Part model, mm, in its own coordinate system. A direction names the side the tool comes from. Round coordinates to 2 decimals unless told otherwise and drop trailing zeros. Write each loop counter-clockwise with the first axis right and the second up, starting at its lowest first coordinate (ties: lowest second). Pieces come first, ordered by that corner, then holes. Notation, with made-up numbers: (-27, -29.75) -> (8, -29.75) arc R25 cw to (8, -14.75) -> close; hole circle Ø1 at (-27, -13). An arc over 180 degrees is marked (long way). Use CSV: the item, a comma, the result in double quotes. Start each with the question number.
(1) Saw through at A-A (z = 4.5). Give the cut face in (x, y).
(2) Which spindle directions (+Z, -Z, +X, -X, +Y, -Y) get a long thin tool onto all of the face, cutting with end or side? Do faces 1 (the flat face through (47.5, -1, -1)), 2 (the flat face through (21, -1, 32.121)). Say none if no direction does.
(3) Saw through at C-C (x = 26). Give the cut face in (y, z).
(4) Two-plate mould, pull along Z, no slides. Class faces 3 (the cylindrical face through (-45.09, -1.48, 45)), 4 (the flat face through (-1, 0, 1)), 5 (the cylindrical face through (-46.6, -1.48, 46.64)): released by +Z, released by -Z, zero draft, split by the parting line, or undercut.
(5) Saw through at D-D (y = -1.1). Count the separate pieces of the cut face and the enclosed holes in it, plus the area to 3 significant figures.
(6) Drop a flat-ended pin along its axis: pin 1 (3 mm diameter, centred on x = 43.95, z = -43.95, fed in from -Y). Give the stop position or say it passes through.
(7) Probe line 1 (X direction, y = -2.6, z = 27); line 2 (Z direction, x = -25.4, y = -2.05); line 3 (Z direction, x = -43.95, y = -1.8). List the from-to ranges inside material, lowest first. Write a range as [from, to].
(8) Saw through at B-B (x = 0). Give the cut face in (y, z).
```python
from build123d import *

# Parameters (mm, degrees)
F0_R     = 1.55
F0_R_2   = 3.8
F0_R_3   = 3
F0_W     = 22.7
F0_H     = 10.2
F1_DEPTH = 3


with BuildPart() as f1:
    # F0 (on Front) → F1 (new body)
    with BuildSketch(Plane.XZ):
        with BuildLine():
            Line((-44.5, -47.5), (44.5, -47.5))
            ThreePointArc((44.5, -47.5), (46.62132, -46.62132), (47.5, -44.5))
            Line((47.5, -44.5), (47.5, 44.5))
            ThreePointArc((47.5, 44.5), (46.62132, 46.62132), (44.5, 47.5))
            Line((44.5, 47.5), (-44.5, 47.5))
            ThreePointArc((-44.5, 47.5), (-46.62132, 46.62132), (-47.5, 44.5))
            Line((-47.5, 44.5), (-47.5, -44.5))
            ThreePointArc((-47.5, -44.5), (-46.62132, -46.62132), (-44.5, -47.5))
        make_face()
        with Locations((-43.95, -43.95)):
            Circle(F0_R, mode=Mode.SUBTRACT)
        with Locations((-25.4, -18.782858)):
            Circle(F0_R_2, mode=Mode.SUBTRACT)
        with Locations((43.95, -43.95)):
            Circle(F0_R, mode=Mode.SUBTRACT)
        with Locations((0, -18.782858)):
            Circle(F0_R_2, mode=Mode.SUBTRACT)
        with Locations((25.4, -18.782858)):
            Circle(F0_R_2, mode=Mode.SUBTRACT)
        with Locations((-21.6, 4.5)):
            Circle(F0_R_3, mode=Mode.SUBTRACT)
        with Locations((-43.95, 43.95)):
            Circle(F0_R, mode=Mode.SUBTRACT)
        with Locations((-21.6, 27.020905)):
            Rectangle(F0_W, F0_H, mode=Mode.SUBTRACT)
        with Locations((21.6, 4.5)):
            Circle(F0_R_3, mode=Mode.SUBTRACT)
        with Locations((21.6, 27.020905)):
            Rectangle(F0_W, F0_H, mode=Mode.SUBTRACT)
        with Locations((43.95, 43.95)):
            Circle(F0_R, mode=Mode.SUBTRACT)
    extrude(amount=F1_DEPTH)


solid = f1.part
```
Answers:
1,outline,"(-47.5, -3) -> (-24.6, -3) -> (-24.6, 0) -> (-47.5, 0) -> close; (-18.6, -3) -> (18.6, -3) -> (18.6, 0) -> (-18.6, 0) -> close; (24.6, -3) -> (47.5, -3) -> (47.5, 0) -> (24.6, 0) -> close"
2,face 1,"+Z, -Z, +X, +Y, -Y"
2,face 2,"+Y, -Y"
3,outline,"(-3, -47.5) -> (0, -47.5) -> (0, -22.54) -> (-3, -22.54) -> close; (-3, -15.03) -> (0, -15.03) -> (0, 21.92) -> (-3, 21.92) -> close; (-3, 32.12) -> (0, 32.12) -> (0, 47.5) -> (-3, 47.5) -> close"
4,face 3,"undercut"
4,face 4,"zero draft"
4,face 5,"released by +Z"
5,separate pieces,"1"
5,enclosed holes,"11"
5,area,"8,330 mm²"
6,pin 1,"passes through"
7,line 1,"x = [-47.5, -32.95], [-10.25, 10.25], [32.95, 47.5]"
7,line 2,"z = [-47.5, -22.58], [-14.98, 21.92], [32.12, 47.5]"
7,line 3,"z = [-47.5, -45.5], [-42.4, 42.4], [45.5, 47.5]"
8,outline,"(-3, -47.5) -> (0, -47.5) -> (0, -22.58) -> (-3, -22.58) -> close; (-3, -14.98) -> (0, -14.98) -> (0, 47.5) -> (-3, 47.5) -> close"
